Autodesk Fusion 360 part; units mm, degrees
sketch "Sketch1" plane through (0, 0, 0) normal (0, 0, 1) x (1, 0, 0)
  line L0 (0, 0) -> (80, 0)
  line L1 (80, 0) -> (80, 170)
  line L2 (80, 170) -> (0, 170)
  line L3 (0, 170) -> (0, 0)
  dimension "d1" = 80
  dimension "d2" = 170
extrude "Extrude1" add sketch "Sketch1" along normal blind 80
sketch "Sketch2" plane through (80, 0, 0) normal (1, 0, 0) x (0, 1, 0)
  line L0 (0, 0) -> (170, 0)
  line L1 (170, 0) -> (170, 80)
  line L2 (170, 80) -> (0, 80)
  line L3 (0, 80) -> (0, 0)
  line L4 (0, 50) -> (10, 50)
  arc A0 (40, 80) -> (10, 50) centre (40, 50) ccw
  line L5 (40, 80) -> (40, 40)
  line L6 (40, 40) -> (140, 40)
  line L7 (140, 40) -> (140, 60)
  line L8 (140, 60) -> (170, 60)
  dimension "d5" = 10
  dimension "d6" = 30
  dimension "d8" = 40
  dimension "d9" = 30
  dimension "d10" = 20
  dimension "d12" = 30
extrude "Extrude2" cut sketch "Sketch2" against normal blind 80 contours L2 L3 L4 A0 | L1 L2 L5 L6 L7 L8
sketch "Sketch3" plane through (0, 170, 0) normal (0, 1, 0) x (-1, 0, 0)
  line L0 (0, 60) -> (-80, 60)
  line L1 (-80, 60) -> (-80, 0)
  line L2 (-80, 0) -> (0, 0)
  line L3 (0, 0) -> (0, 60)
  arc A0 (-20, 60) -> (-60, 60) centre (-40, 60) ccw
  dimension "d15" = 20
extrude "Extrude3" add sketch "Sketch3" against normal blind 30 contours L0 A0
sketch "Sketch4" plane through (0, 0, 0) normal (0, -1, 0) x (1, 0, 0)
  line L0 (80, 50) -> (0, 50)
  line L1 (0, 50) -> (0, 0)
  line L2 (0, 0) -> (80, 0)
  line L3 (80, 0) -> (80, 50)
  line L4 (40, 50) -> (40, -1.5381) construction
  line L5 (20, 0) -> (20, 20)
  line L6 (20, 20) -> (30, 20)
  line L7 (30, 20) -> (30, 40)
  line L8 (30, 40) -> (40, 40)
  line L9 (60, 0) -> (60, 20)
  line L10 (50, 40) -> (40, 40)
  line L11 (60, 20) -> (50, 20)
  line L12 (50, 20) -> (50, 40)
  dimension "d18" = 20
  dimension "d19" = 10
  dimension "d20" = 20
  dimension "d21" = 10
extrude "Extrude4" cut sketch "Sketch4" against normal blind 170 contours L2 L5 L6 L7 L8 L9 L10 L11 L12
sketch "Sketch5" plane through (0, 40, 0) normal (0, 1, 0) x (-1, 0, 0)
  line L0 (-80, 80) -> (-80, 40)
  line L1 (-80, 40) -> (-50, 40)
  line L2 (-50, 40) -> (-30, 40)
  line L3 (-30, 40) -> (0, 40)
  line L4 (0, 40) -> (0, 80)
  line L5 (0, 80) -> (-80, 80)
  line L6 (-50, 40) -> (-50, 50)
  line L7 (-50, 50) -> (-30, 50)
  line L8 (-30, 40) -> (-30, 42.318)
  line L9 (-30, 42.318) -> (-30, 50)
  line L10 (-53.8731, 40) -> (-53.8731, 53.8731)
  line L11 (-53.8731, 53.8731) -> (-26.1269, 53.8731)
  line L12 (-26.1269, 42.318) -> (-26.1269, 53.8731)
  line L13 (-26.1269, 40) -> (-26.1269, 42.318)
  dimension "d24" = 10
  dimension "d25" = -3.8731
extrude "Extrude5" add sketch "Sketch5" along normal blind 100 contours L1 L3 L6 L7 L8 L9 L10 L11 L12 L13
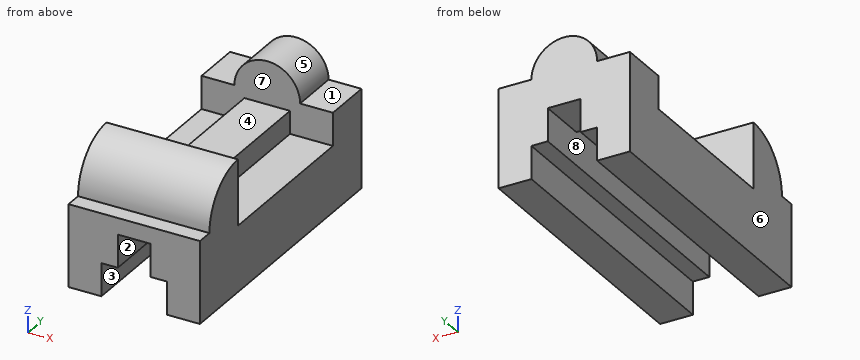
Could you check a few things on this model? Use its own coordinates, in mm. Face numbers are marked on the shaded views. A direction names the side the tool comes from. Round coordinates to 2 decimals unless told otherwise and drop trailing zeros. Order: outer loops, then holes, each group sorted by start corner. A loop starts at its lowest first (then second) coordinate and runs counter-clockwise, first axis right, second up.
(1) Imagine slicing it at A-A (z = 65). Write out the boundary of the cut face in (x, y), plus the area to 3 significant figures.
Response values:
outline: (0, 14.02) - (80, 14.02) - (80, 40) - (0, 40) - close; (20.64, 140) - (59.36, 140) - (59.36, 170) - (20.64, 170) - close
area: 3,240 mm2
(2) Imagine slicing it at C-C (y = 43.5). Write out the boundary of the cut face in (x, z).
Response values:
outline: (0, 0) - (20, 0) - (20, 20) - (30, 20) - (30, 50) - (50, 50) - (50, 20) - (60, 20) - (60, 0) - (80, 0) - (80, 40) - (53.87, 40) - (53.87, 53.87) - (26.13, 53.87) - (26.13, 40) - (0, 40) - close
(3) Imagine slicing it at B-B (x = 40). Write out the boundary of the cut face in (y, z).
Response values:
outline: (0, 40) - (40, 40) - (40, 50) - (140, 50) - (140, 40) - (170, 40) - (170, 80) - (140, 80) - (140, 53.87) - (40, 53.87) - (40, 80) arc R30 ccw to (10, 50) - (0, 50) - close
(4) Which directions (+Z, -Z, +X, -X, +Y, -Y) give clear straight access to the entire face, cutting with the end or side of a thin tool? Please do the marked faces 1, 2, 3, 4 and 5.
Response values:
face 1: +Z, +X, +Y
face 2: -Z
face 3: -Z, +Y, -Y
face 4: +Z, +X, -X
face 5: +Z, +Y
(5) Imagine slicing it at D-D (z = 44.5). Write out the boundary of the cut face in (x, y), plus the area to 3 significant figures.
Response values:
outline: (0, 0) - (80, 0) - (80, 40) - (53.87, 40) - (53.87, 140) - (80, 140) - (80, 170) - (0, 170) - (0, 140) - (26.13, 140) - (26.13, 40) - (0, 40) - close; hole (30, 40) - (50, 40) - (50, 140) - (30, 140) - close
area: 6,370 mm2
(6) Please list where these lines run through material, in increasing order: line 1 along X through (y, z) = (90, 12); line 2 along X through (y, z) = (106.5, 25); line 3 along Y through (x, z) = (48, 49).
Response values:
line 1: x = 0 to 20, 60 to 80
line 2: x = 0 to 30, 50 to 80
line 3: y = 0 to 40, 140 to 170
(7) I'm going to push flat-ended pins straight in: pin 1 (5 mm diameter, centred on x = 8, y = 98, fed in from +Z); pin 2 (8 mm diameter, centred on x = 25, y = 52.5, fed in from -Z); pin 3 (10 mm diameter, centred on x = 39, y = 152, fed in from -Z). Where does each tip first touch, or does it pass through?
Response values:
pin 1: stops at z = 40
pin 2: stops at z = 20
pin 3: stops at z = 40
(8) If we mould it in two halves opening along X, with no side actions, what happens to the marked faces 6, 7 and 8? For each: released by +X, released by -X, zero draft, split by the parting line, or undercut.
Response values:
face 6: released by -X
face 7: zero draft
face 8: undercut
